Geometry check sheet. Reference: drawing and pictorial views, mm from the part's lowest x, y, z. Coordinates: 2 decimals unless noted, no trailing zeros. Loops run counter-clockwise (first coordinate to the right, second up) from the corner with the lowest first, then second, coordinate; pieces in that order, holes last. Notation, with made-up numbers: (-1.75, 78) -> (6.25, 78) arc R21 cw to (6.25, 93) -> close; hole circle Ø7 at (16.25, 51). An arc over 180 degrees is marked (long way). Answer as a JSON object with one key per item and string values. Group by question number.
Q1. Gauge pin test, flat ends, axial feed: pin 1 Ø10 at (y, z) = (12, 25.5) entering from +X; pin 2 Ø4 at (y, z) = (90, 10.5) entering from +X; pin 3 Ø10 at (x, y) = (19, 17.5) entering from +Z; pin 4 Ø4 at (x, z) = (17.5, 36) entering from +Y (3 decimals). Record the tip position at first contact, or that the pin passes through.
Q2. Cross-section at B-B on y = 50. Record the boundary of the cut face in (x, z).
Q3. Cross-section at C-C on x = 16.25. Record the boundary of the cut face in (y, z).
Q4. Cross-section at A-A on x = 2.5. Record the boundary of the cut face in (y, z).
Q5. Release check for a two-part mould opening along Y. For the marked faces 1, 2 and 3 record: released by +Y, released by -Y, zero draft, split by the parting line, or undercut.
Q6. Scan lines: L1, parallel to Y at x = 1, z = 19; L2, parallel to Y at x = 13.25, z = 19.5; L3, parallel to Z at x = 23.5, y = 31. Record each from-to range of solid material in increasing order.
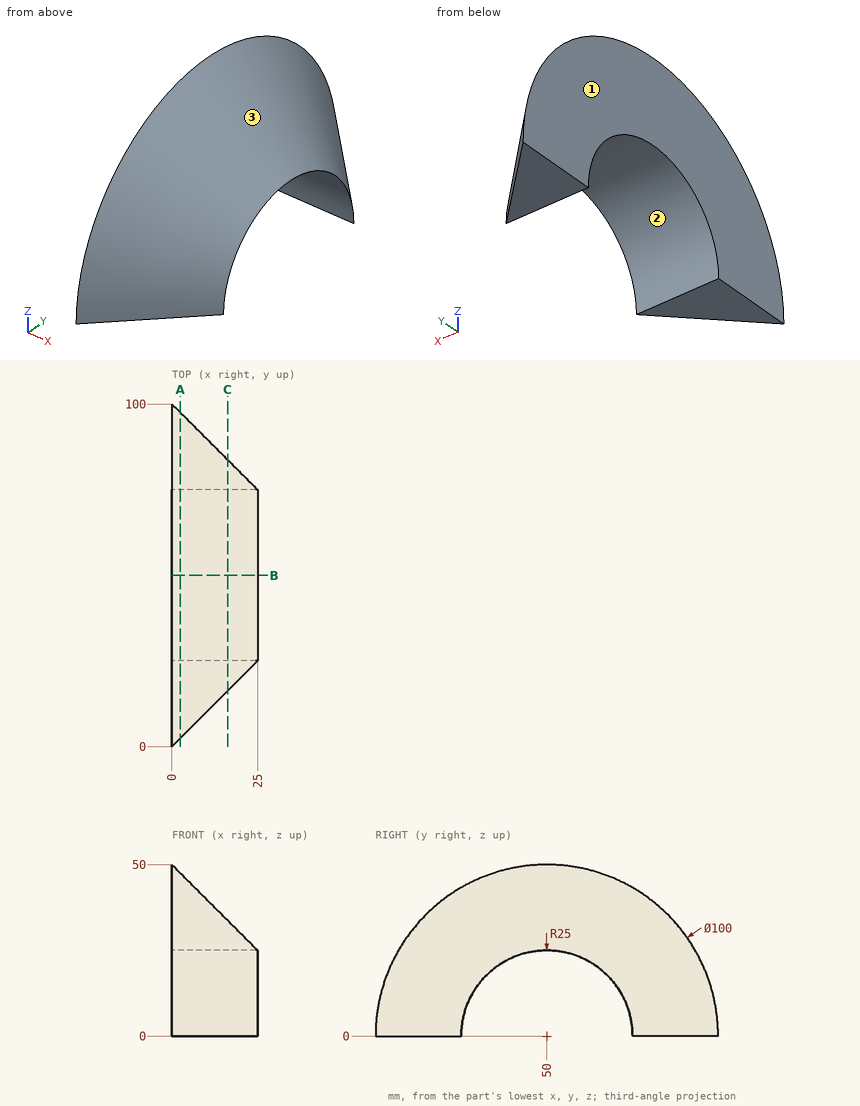
Computed values:
{
 "1": {"pin 1": "stops at x = 9.24", "pin 2": "stops at x = 10.64", "pin 3": "stops at z = 18.85", "pin 4": "passes through"},
 "2": {"outline": "(0, 25) -> (25, 25) -> (0, 50) -> close"},
 "3": {"outline": "(16.25, 0) -> (25, 0) arc R25 cw to (75, 0) -> (83.75, 0) arc R33.75 ccw to start"},
 "4": {"outline": "(2.5, 0) -> (25, 0) arc R25 cw to (75, 0) -> (97.5, 0) arc R47.5 ccw to start"},
 "5": {"face 1": "zero draft", "face 2": "undercut", "face 3": "split by the parting line"},
 "6": {"L1": "y = 4.83 to 33.75, 66.25 to 95.17", "L2": "y = 18.85 to 34.36, 65.64 to 81.15", "L3": "z = 16.25 to 18.47"}
}
